Can you work these out from the model? Positions are in its coordinate system, mm. A direction names the side the tool comes from. Round coordinates to 2 decimals unless told otherwise and drop trailing zeros. Order: outer loops, then holes, each group sorted by start corner. A loop starts at its lowest first (then second) coordinate and runs counter-clockwise, first axis right, second up.
Q1. For faces 4 (the face through (-0.07, -1.4, 2.94)), 5 (the face through (6.785, 1.507, 18.254)), 6 (the face through (0, 0.3, 1)), 7 (the face through (1.1, 1.5, -10.5)), 8 (the face through (-1.602, -4.021, 18.332)), which set-ups out of +Z, -Z, +X, -X, +Y, -Y let a thin tool reach every point of the face, with its end or its side?
Q2. If I drill on line 1 (Y direction, x = -0.75, z = 8); line 2 (Z direction, x = 0, y = -0.25); line 3 (Y direction, x = -4.75, z = 2.5), over which ranges is the centre line in solid material (lowest first)?
Q3. If we section it at A-A (z = 8): Please give me the cut outline in (x, y).
Q4. We'd pull the mould along X, two halves only. Please class faces 1 (the face through (-0.571, 1.188, 18.332)), 2 (the face through (3.62, 4.72, 4.15)), 3 (the face through (0, -0.3, 1)): pulls with the +X half, pulls with the -X half, needs draft (parallel to the pull), parting line crosses it, or undercut.
Q5. If we section it at B-B (y = 0): Please give me the cut outline in (x, z).
Q6. If we section it at C-C (x = 0): Count the separate pieces of the cut face and the enclosed holes in it, plus the area to 3 significant figures.
Q7. Will these pins go through, and if not, where does the flat tip stop? P1, Ø6, axis at x = -5, z = 17.5, coming from the +Y side; P2, Ø1.5, axis at y = -1, z = 10.5, coming from the -X side; P3, Ø5, axis at y = 1, z = 10.5, coming from the -X side; P4, Ø4, axis at x = -3, y = -0.5, coming from the -Z side.
from build123d import *

# Parameters (mm, degrees)
SKETCH014_R             = 7.05
PAD004_DEPTH            = 2.5
SKETCH015_R             = 6.95
PAD005_DEPTH            = 0.5
SKETCH016_R             = 5.95
PAD006_DEPTH            = 28.5
SKETCH018_R             = 1.9
POCKET010_DEPTH         = 5
SKETCH019_R             = 1.6
POCKET011_DEPTH         = 31.501
SKETCH020_W             = 0.6
SKETCH020_H             = 16
POCKET012_DEPTH         = 34
CHAMFER_SIZE            = 0.4
CHAMFER003_SIZE         = 0.4
BODY003_ROLL_ANGLE      = 180
BODY003_PLACEMENT_ANGLE = -90


with BuildPart() as part:
    # Sketch014 → Pad004 (new body)
    with BuildSketch(Plane.XY):
        Circle(SKETCH014_R)
    extrude(amount=PAD004_DEPTH)

    # Sketch015 (on DatumPlane) → Pad005 (join)
    with BuildSketch(Plane.XY.offset(2.5)):
        Circle(SKETCH015_R)
    extrude(amount=PAD005_DEPTH)

    # Sketch016 (on DatumPlane) → Pad006 (join)
    with BuildSketch(Plane.XY.offset(3)):
        Circle(SKETCH016_R)
    extrude(amount=PAD006_DEPTH)

    # Sketch018 (on DatumPlane) → Pocket010 (cut)
    with BuildSketch(Plane.XY):
        with Locations((-3, 0)):
            Circle(SKETCH018_R)
        with Locations((3, 0)):
            Circle(SKETCH018_R)
    extrude(amount=POCKET010_DEPTH, mode=Mode.SUBTRACT)

    # Sketch019 (on DatumPlane) → Pocket011 (cut, through all)
    with BuildSketch(Plane.XY):
        with Locations((-3, 0)):
            Circle(SKETCH019_R)
        with Locations((3, 0)):
            Circle(SKETCH019_R)
    extrude(amount=POCKET011_DEPTH, mode=Mode.SUBTRACT)

    # Sketch020 (on DatumPlane) → Pocket012 (cut)
    with BuildSketch(Plane.XY.offset(43)):
        Rectangle(SKETCH020_W, SKETCH020_H)
    extrude(amount=-POCKET012_DEPTH, mode=Mode.SUBTRACT)

    # Chamfer
    chamfer_edges = [part.edges().sort_by_distance(p)[0] for p in [
        (-0.3, 0, 31.5),
        (-5.95, 0, 31.5),
        (0.3, 0, 31.5),
        (4.312047, -4.099848, 31.5),
        (4.312047, 4.099848, 31.5),
    ]]
    chamfer(chamfer_edges, length=CHAMFER_SIZE)

    # Chamfer003
    chamfer003_edges = [part.edges().sort_by_distance(p)[0] for p in [
        (-7.05, 0, 0),
        (-4.9, 0, 0),
        (1.1, 0, 0),
    ]]
    chamfer(chamfer003_edges, length=CHAMFER003_SIZE)


with BuildPart() as part_1:
    # Body003 roll: moved
    add(part.part.rotate(Axis((0, 0, 0), (1, 0, 0)), BODY003_ROLL_ANGLE))


with BuildPart() as part_2:
    # Body003 placement: moved
    add(part_1.part.moved(Location((0, 0, 21))).rotate(Axis((0, 0, 21), (0, 0, 1)), BODY003_PLACEMENT_ANGLE))


solid = part_2.part
Solution:
1. face 4: +Z, -Z
1. face 5: -Z
1. face 6: -Z, +X, -X
1. face 7: -Z, +X, -X, +Y, -Y
1. face 8: +Z
2. line 1: y = -5.9 to -4.41, -1.59 to -0.3, 0.3 to 1.59, 4.41 to 5.9
2. line 2: z = 12 to 21
2. line 3: y = -3.58 to -0.3, 0.3 to 3.58
3. outline: (-5.94, -0.3) arc R5.95 ccw to (5.94, -0.3) - close; (-5.94, 0.3) - (5.94, 0.3) arc R5.95 ccw to start; hole circle Ø3.2 at (0, -3); hole circle Ø3.2 at (0, 3)
4. face 1: undercut
4. face 2: parting line crosses it
4. face 3: needs draft
5. outline: (-7.05, 18.5) - (-6.95, 18.5) - (-6.95, 18) - (-5.95, 18) - (-5.95, 12) - (5.95, 12) - (5.95, 18) - (6.95, 18) - (6.95, 18.5) - (7.05, 18.5) - (7.05, 20.6) - (6.65, 21) - (-6.65, 21) - (-7.05, 20.6) - close
6. separate pieces: 3
6. enclosed holes: 0
6. area: 159 mm2
7. P1: stops at y = 6.71
7. P2: stops at x = -5.94
7. P3: stops at x = -5.95
7. P4: stops at z = -10.5
